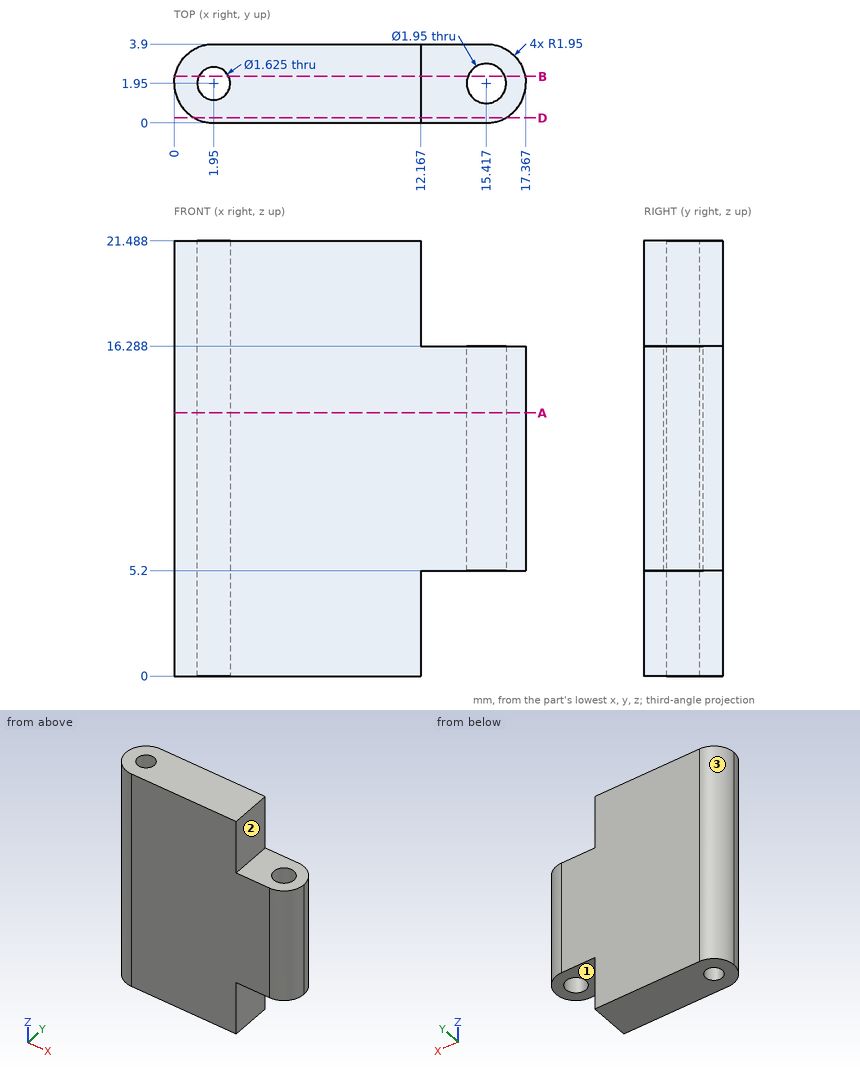
Geometry check sheet. Reference: drawing and pictorial views, mm from the part's lowest x, y, z. A direction names the side the tool comes from. Coordinates: 2 decimals unless noted, no trailing zeros. Order: outer loops, then holes, each group sorted by start corner. A loop starts at its lowest first (then second) coordinate and runs counter-clockwise, first axis right, second up. Notation, with made-up numbers: (44.5, -20) -> (67.5, -20) arc R32 ccw to (67.5, 9) -> close; hole circle Ø6 at (52, -33.5). An arc over 180 degrees is marked (long way). Write item = value, one per line. Start each with the question number.
1) Access from +Z, -Z, +X, -X, +Y, -Y to the whole of each face (thin tool, end or side, straight path). Record for the marked faces 1, 2 and 3.
2) Go/stop test with flat-tipped pins: P1, Ø1.2, axis at x = 15, y = 1.5, coming from the +Z side; P2, Ø2, axis at y = 2.5, z = 3.5, coming from the +X side. Record where each tip stops, or that it passes through.
3) Material ranges on L1, parallel to Y at x = 1.95, z = 13.25; L2, parallel to X at y = 2.5, z = 14; L3, parallel to Z at x = 14.5, y = 0.8, recorded low to high.
4) Cross-section at A-A (z = 13). State how many separate pieces and enclosed holes the cut face has, then the cut area to 3 significant figures.
5) Cross-section at D-D (y = 0.25). Enter the section's corners in (x, z) (1 decimal), then the cut area to 3 significant figures.
6) Cross-section at B-B (y = 2.3). Enter the section's corners in (x, z) (1 decimal), then the cut area to 3 significant figures.
Ans:
q1.face_1 = -Z, +X, +Y, -Y
q1.face_2 = +Z, +X, +Y, -Y
q1.face_3 = +Z, -Z, -X, +Y
q2.P1 = 16.29
q2.P2 = 12.17
q3.L1 = 0 to 1.14, 2.76 to 3.9
q3.L2 = 0.08 to 1.35, 2.55 to 14.61, 16.22 to 17.29
q3.L3 = 5.2 to 16.29
q4.separate_pieces = 1
q4.enclosed_holes = 2
q4.area = 59.4 mm²
q5.outline = (1, 0) -> (12.2, 0) -> (12.2, 5.2) -> (16.4, 5.2) -> (16.4, 16.3) -> (12.2, 16.3) -> (12.2, 21.5) -> (1, 21.5) -> close
q5.area = 287 mm²
q6.outline = (0, 0) -> (1.2, 0) -> (1.2, 21.5) -> (0, 21.5) -> close; (2.7, 0) -> (12.2, 0) -> (12.2, 5.2) -> (14.5, 5.2) -> (14.5, 16.3) -> (12.2, 16.3) -> (12.2, 21.5) -> (2.7, 21.5) -> close; (16.3, 5.2) -> (17.3, 5.2) -> (17.3, 16.3) -> (16.3, 16.3) -> close
q6.area = 266 mm²
